Can you work these out from the drawing? Everything is in mm from the part's minimum corner. A direction names the side the tool comes from. Coordinates: 2 decimals unless noted, no trailing zeros. Loops run counter-clockwise (first coordinate to the right, second up) from the corner with the lowest first, then second, coordinate; pieces in that order, holes last. Notation, with made-up numbers: (89.25, 81) - (133.25, 81) arc R31 cw to (133.25, 116) - close; hole circle Ø3 at (50.5, 70). An arc over 180 degrees is marked (long way). One line per question, with ' | ' between items. Start each with the question number.
1. I want a section at A-A, the plane z = 533. Write out the boundary of the cut face in (x, y), then the cut area to 3 significant figures.
2. Please list where these lines run through material, in increasing order: L1, parallel to Z at x = 629, y = 76; L2, parallel to Z at x = 40, y = 76; L3, parallel to X at y = 83, z = 541.5. Write a range as [from, to].
3. I want a section at C-C, the plane y = 137. Write out the boundary of the cut face in (x, z), then the cut area to 3 significant figures.
4. We'd pull the mould along X, two halves only. Please class the marked faces 1, 2 and 3: pulls with the +X half, pulls with the -X half, needs draft (parallel to the pull), parting line crosses it, or undercut.
5. I want a section at D-D, the plane x = 145. Write out the boundary of the cut face in (y, z), then the cut area to 3 significant figures.
6. I want a section at B-B, the plane y = 201.5. Write out the boundary of the cut face in (x, z).
7. Which directions (+Z, -Z, +X, -X, +Y, -Y) give clear straight access to the entire face, cutting with the end or side of a thin tool? Please do the marked faces 4, 5 and 6.
8. I'm going to push a flat-ended pin straight in: P1, Ø5, axis at x = 536.5, z = 744, coming from the +Y side. Where does the tip first touch, or does it pass through?
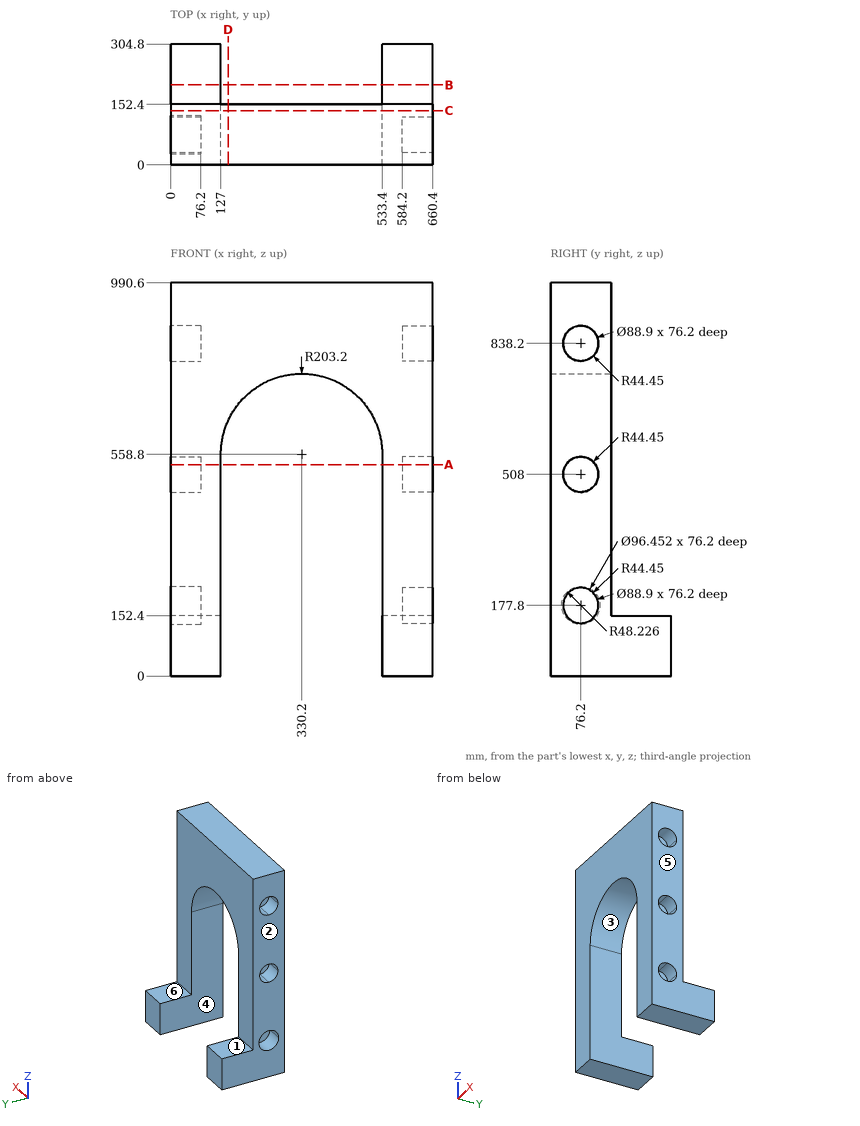
Results are:
1) outline: (0, 0) - (127, 0) - (127, 152.4) - (0, 152.4) - (0, 112.95) - (76.2, 112.95) - (76.2, 39.45) - (0, 39.45) - close; (533.4, 0) - (660.4, 0) - (660.4, 39.45) - (584.2, 39.45) - (584.2, 112.95) - (660.4, 112.95) - (660.4, 152.4) - (533.4, 152.4) - close | area: 27,500 mm2
2) L1: z = [0, 133.35], [222.25, 463.55], [552.45, 793.75], [882.65, 990.6] | L2: z = [0, 129.57], [226.03, 463.55], [552.45, 793.75], [882.65, 990.6] | L3: x = [76.2, 127], [533.4, 584.2]
3) outline: (0, 0) - (127, 0) - (127, 558.8) arc R203.2 cw to (533.4, 558.8) - (533.4, 0) - (660.4, 0) - (660.4, 990.6) - (0, 990.6) - close | area: 362,000 mm2
4) face 1: needs draft | face 2: pulls with the -X half | face 3: undercut
5) outline: (0, 642.41) - (152.4, 642.41) - (152.4, 990.6) - (0, 990.6) - close | area: 53,100 mm2
6) outline: (0, 0) - (127, 0) - (127, 152.4) - (0, 152.4) - close; (533.4, 0) - (660.4, 0) - (660.4, 152.4) - (533.4, 152.4) - close
7) face 4: -Z, +Y, -Y | face 5: +Z, -Z, +X, +Y, -Y | face 6: +Z, +X, -X, +Y
8) P1: stops at y = 152.4
